```python
from build123d import *

# Parameters (mm, degrees)
EXTRUDE_2_DEPTH     = 5
SKETCH_3_R          = 1.6
CUT_EXTRUDE_1_DEPTH = 172.275363085
SKETCH_4_W          = 164.707045146
SKETCH_4_H          = 1
CUT_EXTRUDE_2_DEPTH = 172.275363085
EXTRUDE_3_DEPTH     = 5


with BuildPart() as part:
    # 草图2 → 凸台-拉伸2 (new body)
    with BuildSketch(Plane.XY):
        Polygon((0, 0), (112.5, 0), (137.5, 102), (-25, 102), align=None)
    extrude(amount=EXTRUDE_2_DEPTH)

    # 草图3 → 切除-拉伸1 (cut, through all)
    with BuildSketch(Plane.XY.offset(5)):
        with Locations((-18.234733944, 87)):
            Circle(SKETCH_3_R)
        with Locations((113.087675121, 15)):
            Circle(SKETCH_3_R)
        with Locations((-0.587675121, 15)):
            Circle(SKETCH_3_R)
        with Locations((130.734733944, 87)):
            Circle(SKETCH_3_R)
    extrude(amount=-CUT_EXTRUDE_1_DEPTH, mode=Mode.SUBTRACT)

    # 草图4 → 切除-拉伸2 (cut, through all)
    with BuildSketch(Plane.XY.offset(5)):
        with Locations((57.353522573, 101.5)):
            Rectangle(SKETCH_4_W, SKETCH_4_H)
    extrude(amount=-CUT_EXTRUDE_2_DEPTH, mode=Mode.SUBTRACT)

    # 草图5 → 凸台-拉伸3 (add)
    with BuildSketch(Plane.XY.offset(5)):
        Polygon((0, 0), (0.980392157, -4), (111.519607843, -4), (112.5, 0), align=None)
    extrude(amount=-EXTRUDE_3_DEPTH)


solid = part.part
```
The listing builds one solid part. Answer for the finished solid, in the listing's coordinates (mm). Give positions to 0.01 mm unless a question says otherwise; leave off trailing zeros. Loops run counter-clockwise (first coordinate to the right, second up) from the corner with the lowest first, then second, coordinate; pieces in that order, holes last. Notation, with made-up numbers: M 22.5,2.25 L 39.5,2.25 A18 ccw 39.5,29.25 Z; hole C -1,7.5 d1. An arc over 180 degrees is marked long. One line per item, written item: value.
Q1. A cutting plane is placed at A-A on z = 1.8. Determine the outline of the cut face in (x, y), then the cut area to 3 significant figures.
Working result:
outline: M -24.75,101 L 0.98,-4 L 111.52,-4 L 137.25,101 Z; hole C -18.23,87 d3.2; hole C -0.59,15 d3.2; hole C 113.09,15 d3.2; hole C 130.73,87 d3.2
area: 14,300 mm^2
Q2. Flat-ended cylindrical pins translate along their axes: P1, Ø3, axis at x = -0.59, y = 15, coming from the +Z side; P2, Ø3, axis at y = 36, z = 2.5, coming from the -X side; P3, Ø3, axis at y = 68, z = 2.5, coming from the -X side. Find the tip coordinate at first contact, or state that the pin passes through.
Working result:
P1: passes through
P2: stops at x = -9.19
P3: stops at x = -17.03
Q3. Find the intervals of material crossed by line 1 (X direction, y = 87, z = 1.45); line 2 (X direction, y = 86, z = 2.95); line 3 (X direction, y = 39.5, z = 1.95), in increasing order. Write a range as from..to.
Working result:
line 1: x = -21.32..-19.83, -16.63..129.13, 132.33..133.82
line 2: x = -21.08..-19.48, -16.99..129.49, 131.98..133.58
line 3: x = -9.68..122.18
Q4. A cutting plane is placed at D-D on x = -13. Determine the outline of the cut face in (y, z), then the cut area to 3 significant figures.
Working result:
outline: M 53.04,0 L 101,0 L 101,5 L 53.04,5 Z
area: 240 mm^2
Q5. Determine the mould class of faces 1 (the face through (55, 49, 0)), 2 (the face through (55, -4, 3)), 3 (the face through (114.614, 15.481, 2.535)) for opening direction Y: +Y half, -Y half, draft (parallel to the pull), parting line (faces both ways), or undercut.
Working result:
face 1: draft
face 2: -Y half
face 3: undercut
Q6. A cutting plane is placed at C-C on y = 15. Determine the outline of the cut face in (x, z).
Working result:
outline: M -3.68,0 L -2.19,0 L -2.19,5 L -3.68,5 Z; M 1.01,0 L 111.49,0 L 111.49,5 L 1.01,5 Z; M 114.69,0 L 116.18,0 L 116.18,5 L 114.69,5 Z
Q7. A cutting plane is placed at B-B on y = 87. Determine the outline of the cut face in (x, z), then the cut area to 3 significant figures.
Working result:
outline: M -21.32,0 L -19.83,0 L -19.83,5 L -21.32,5 Z; M -16.63,0 L 129.13,0 L 129.13,5 L -16.63,5 Z; M 132.33,0 L 133.82,0 L 133.82,5 L 132.33,5 Z
area: 744 mm^2
